Could you check a few things on this model? Use its own coordinates, in mm. Face numbers are marked on the shaded views. A direction names the side the tool comes from. Give positions to 0.01 mm unless a question says otherwise; leave off trailing zeros. Order: outer loops, then holes, each group sorted by start corner. A loop starts at its lowest first (then second) coordinate and runs counter-clockwise, first axis right, second up. Notation, with made-up numbers: (45, 59) - (86, 59) arc R10 ccw to (86, 65) - close; hole circle Ø2 at (24.5, 53.25). An arc over 180 degrees is marked (long way). One line per question, with ' | ' between items. Start each with the question number.
1. Imagine slicing it at C-C (z = 3). Please give me the cut outline in (x, y), and give its area (3 significant figures).
2. Imagine slicing it at D-D (x = 7.25). Please give me the cut outline in (y, z), and give its area (3 significant figures).
3. Imagine slicing it at B-B (x = -0.75). Please give me the cut outline in (y, z), and give its area (3 significant figures).
4. Which directions (+Z, -Z, +X, -X, +Y, -Y) give clear straight access to the entire face, cutting with the end or side of a thin tool? Please do the marked faces 4, 5 and 6.
5. I need wall thicknesses on probe 1 along Y at (x, z) = (-0.75, 0.65); probe 2 along Z at (x, y) = (9.5, 8.5); probe 3 along Y at (x, z) = (10.75, 3.9). Which ranges of each line are inside material? Lowest first, please. Write a range as from..to.
6. For P1, Ø1.2, axis at y = 1.5, z = 0.5, coming from the +X side; P2, Ø3, axis at x = 10, z = 3, coming from the -Y side; P3, Ø6.5, axis at x = 2.5, y = -4.5, coming from the +Z side, each with a flat end and sliding along its axis, tell me the tip position at first contact or that it passes through.
7. If we mould it in two halves opening along X, with no side actions, what happens to the marked faces 1, 2 and 3? For each: released by +X, released by -X, zero draft, split by the parting line, or undercut.
8. Imagine slicing it at A-A (y = -6.75). Please give me the cut outline in (x, z).
```python
from build123d import *

# Parameters (mm, degrees)
SKETCH_1_W          = 13
SKETCH_1_H          = 25
SKETCH_1_R          = 2.25
EXTRUDE_1_DEPTH     = 1.5
SKETCH_2_R          = 3
SKETCH_2_R_2        = 1.5
EXTRUDE_2_DEPTH     = 25
SKETCH_3_W          = 3
SKETCH_3_H          = 25
EXTRUDE_3_DEPTH     = 1.5
SKETCH_4_W          = 6
SKETCH_4_H          = 6.25
CUT_EXTRUDE_1_DEPTH = 7


with BuildPart() as part:
    # Sketch 1 → Extrude 1 (new body)
    with BuildSketch(Plane.XY):
        Rectangle(SKETCH_1_W, SKETCH_1_H)
        with Locations((-0.75, 6.75)):
            Circle(SKETCH_1_R, mode=Mode.SUBTRACT)
        with Locations((-0.75, -6.75)):
            Circle(SKETCH_1_R, mode=Mode.SUBTRACT)
    extrude(amount=EXTRUDE_1_DEPTH)



with BuildPart() as body_2:
    # Sketch 2 → Extrude 2 (new body)
    with BuildSketch(Plane.XZ.offset(12.5)):
        with Locations((9.5, 3)):
            Circle(SKETCH_2_R)
        with Locations((9.5, 3)):
            Circle(SKETCH_2_R_2, mode=Mode.SUBTRACT)
    extrude(amount=-EXTRUDE_2_DEPTH)


with BuildPart() as part_1:
    add(part.part)

    add(body_2.part)  # Extrude 3 merges body 2
    # Sketch 3 → Extrude 3 (add)
    with BuildSketch(Plane(origin=(0, 0, 0), x_dir=(-1, 0, 0), z_dir=(0, 0, -1))):
        with Locations((-8, 0)):
            Rectangle(SKETCH_3_W, SKETCH_3_H)
    extrude(amount=-EXTRUDE_3_DEPTH)

    # Sketch 4 → Cut-Extrude 1 (cut, through all)
    with BuildSketch(Plane(origin=(0, 0, 0), x_dir=(-1, 0, 0), z_dir=(0, 0, -1))):
        with Locations((-9.5, -9.375)):
            Rectangle(SKETCH_4_W, SKETCH_4_H)
        with Locations((-9.5, 3.125)):
            Rectangle(SKETCH_4_W, SKETCH_4_H)
    extrude(amount=-CUT_EXTRUDE_1_DEPTH, mode=Mode.SUBTRACT)


solid = part_1.part
```
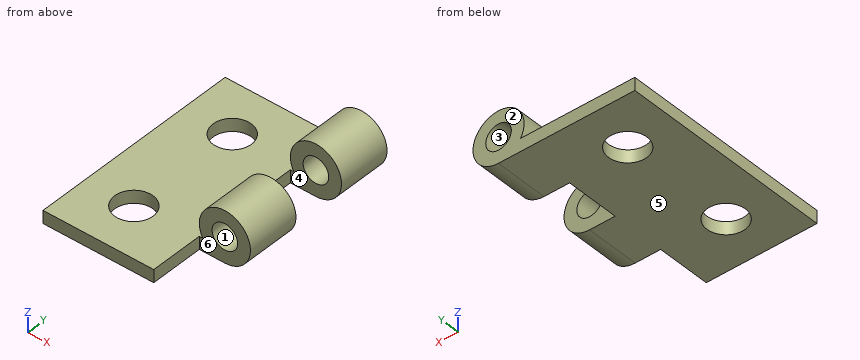
Results found:
1) outline: (6.5, -6.25) - (8, -6.25) - (8, 0) - (6.5, 0) - close; (6.5, 6.25) - (8, 6.25) - (8, 12.5) - (6.5, 12.5) - close; (11, -6.25) - (12.5, -6.25) - (12.5, 0) - (11, 0) - close; (11, 6.25) - (12.5, 6.25) - (12.5, 12.5) - (11, 12.5) - close | area: 37.5 mm2
2) outline: (-6.25, 0) - (0, 0) - (0, 4.98) - (-6.25, 4.98) - close; (6.25, 0) - (12.5, 0) - (12.5, 4.98) - (6.25, 4.98) - close | area: 62.3 mm2
3) outline: (-12.5, 0) - (-9, 0) - (-9, 1.5) - (-12.5, 1.5) - close; (-4.5, 0) - (4.5, 0) - (4.5, 1.5) - (-4.5, 1.5) - close; (9, 0) - (12.5, 0) - (12.5, 1.5) - (9, 1.5) - close | area: 24.0 mm2
4) face 4: +Z, -Z, +X | face 5: -Z, +X, -X, +Y, -Y | face 6: +Z, -Z, +X, -Y
5) probe 1: y = -12.5..-9, -4.5..4.5, 9..12.5 | probe 2: z = 0..1.5, 4.5..6 | probe 3: y = -6.25..0, 6.25..12.5
6) P1: stops at x = 6.5 | P2: stops at y = -6.25 | P3: stops at z = 1.5
7) face 1: undercut | face 2: zero draft | face 3: undercut
8) outline: (-6.5, 0) - (-3, 0) - (-3, 1.5) - (-6.5, 1.5) - close; (1.5, 0) - (6.5, 0) - (6.5, 1.5) - (1.5, 1.5) - close
